Can you work these out from the model? Positions are in its coordinate system, mm. Give positions to 0.01 mm unless a question says otherwise; leave off trailing zeros. Order: outer loops, then holes, each group sorted by start corner. A loop starts at its lowest first (then second) coordinate and runs counter-clockwise, first axis right, second up.
Item 1: I'm going to push a flat-ended pin straight in: pin 1 Ø1 at (x, y) = (4, 6) entering from -Z. Where does the tip first touch, or does it pass through?
Item 2: I want a section at A-A, the plane x = 0. Write out the boundary of the cut face in (y, z), then the cut area to 3 significant figures.
Item 3: If I drill on line 1 along Y through (x, z) = (8.5, 70); line 2 along X through (y, z) = (-7.25, -12); line 3 along X through (y, z) = (-4.75, -23), over which ranges is the centre line in solid material (lowest first)?
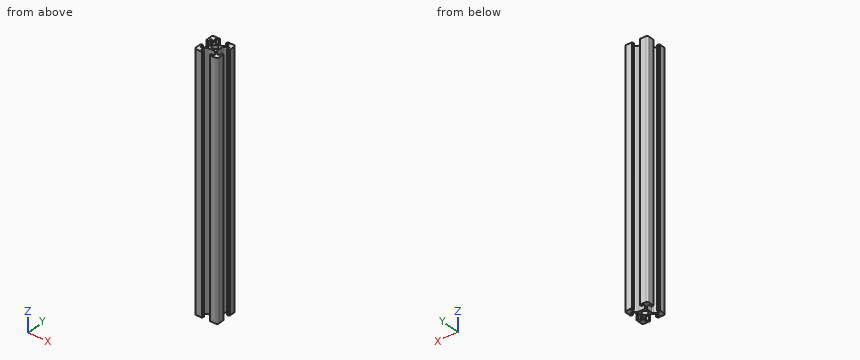
```python
from build123d import *

# Parameters (mm, degrees)
CROQUIS1_R              = 2.5
SALIENTE_EXTRUIR1_DEPTH = 110


with BuildPart() as part:
    # Croquis1 → Saliente-Extruir1 (new, symmetric)
    with BuildSketch(Plane.XY):
        with BuildLine():
            Line((-4.485786438, -3.6372583), (-6.6, -5.751471863))
            Line((-6.6, -5.751471863), (-8.2, -5.751471863))
            Line((-8.2, -5.751471863), (-8.2, -3.1))
            Line((-8.2, -3.1), (-9.5, -3.1))
            Line((-9.5, -3.1), (-9.5, -3.4))
            ThreePointArc((-9.5, -3.4), (-9.558578644, -3.541421356), (-9.7, -3.6))
            Line((-9.7, -3.6), (-10, -3.6))
            Line((-10, -3.6), (-10, -8.5))
            ThreePointArc((-10, -8.5), (-9.560660172, -9.560660172), (-8.5, -10))
            Line((-8.5, -10), (-3.6, -10))
            Line((-3.6, -10), (-3.6, -9.7))
            ThreePointArc((-3.6, -9.7), (-3.541421356, -9.558578644), (-3.4, -9.5))
            Line((-3.4, -9.5), (-3.1, -9.5))
            Line((-3.1, -9.5), (-3.1, -8.2))
            Line((-3.1, -8.2), (-5.751471863, -8.2))
            Line((-5.751471863, -8.2), (-5.751471863, -6.6))
            Line((-5.751471863, -6.6), (-3.6372583, -4.485786438))
            ThreePointArc((-3.6372583, -4.485786438), (-2.988411603, -4.052240935), (-2.223044738, -3.9))
            Line((-2.223044738, -3.9), (2.223044738, -3.9))
            ThreePointArc((2.223044738, -3.9), (2.988411603, -4.052240935), (3.6372583, -4.485786438))
            Line((3.6372583, -4.485786438), (5.751471863, -6.6))
            Line((5.751471863, -6.6), (5.751471863, -8.2))
            Line((5.751471863, -8.2), (3.1, -8.2))
            Line((3.1, -8.2), (3.1, -9.5))
            Line((3.1, -9.5), (3.4, -9.5))
            ThreePointArc((3.4, -9.5), (3.541421356, -9.558578644), (3.6, -9.7))
            Line((3.6, -9.7), (3.6, -10))
            Line((3.6, -10), (8.5, -10))
            ThreePointArc((8.5, -10), (9.560660172, -9.560660172), (10, -8.5))
            Line((10, -8.5), (10, -3.6))
            Line((10, -3.6), (9.7, -3.6))
            ThreePointArc((9.7, -3.6), (9.558578644, -3.541421356), (9.5, -3.4))
            Line((9.5, -3.4), (9.5, -3.1))
            Line((9.5, -3.1), (8.2, -3.1))
            Line((8.2, -3.1), (8.2, -5.751471863))
            Line((8.2, -5.751471863), (6.6, -5.751471863))
            Line((6.6, -5.751471863), (4.485786438, -3.6372583))
            ThreePointArc((4.485786438, -3.6372583), (4.052240935, -2.988411603), (3.9, -2.223044738))
            Line((3.9, -2.223044738), (3.9, 2.223044738))
            ThreePointArc((3.9, 2.223044738), (4.052240935, 2.988411603), (4.485786438, 3.6372583))
            Line((4.485786438, 3.6372583), (6.6, 5.751471863))
            Line((6.6, 5.751471863), (8.2, 5.751471863))
            Line((8.2, 5.751471863), (8.2, 3.1))
            Line((8.2, 3.1), (9.5, 3.1))
            Line((9.5, 3.1), (9.5, 3.4))
            ThreePointArc((9.5, 3.4), (9.558578644, 3.541421356), (9.7, 3.6))
            Line((9.7, 3.6), (10, 3.6))
            Line((10, 3.6), (10, 8.5))
            ThreePointArc((10, 8.5), (9.560660172, 9.560660172), (8.5, 10))
            Line((8.5, 10), (3.6, 10))
            Line((3.6, 10), (3.6, 9.7))
            ThreePointArc((3.6, 9.7), (3.541421356, 9.558578644), (3.4, 9.5))
            Line((3.4, 9.5), (3.1, 9.5))
            Line((3.1, 9.5), (3.1, 8.2))
            Line((3.1, 8.2), (5.751471863, 8.2))
            Line((5.751471863, 8.2), (5.751471863, 6.6))
            Line((5.751471863, 6.6), (3.6372583, 4.485786438))
            ThreePointArc((3.6372583, 4.485786438), (2.988411603, 4.052240935), (2.223044738, 3.9))
            Line((2.223044738, 3.9), (-2.223044738, 3.9))
            ThreePointArc((-2.223044738, 3.9), (-2.988411603, 4.052240935), (-3.6372583, 4.485786438))
            Line((-3.6372583, 4.485786438), (-5.751471863, 6.6))
            Line((-5.751471863, 6.6), (-5.751471863, 8.2))
            Line((-5.751471863, 8.2), (-3.1, 8.2))
            Line((-3.1, 8.2), (-3.1, 9.5))
            Line((-3.1, 9.5), (-3.4, 9.5))
            ThreePointArc((-3.4, 9.5), (-3.541421356, 9.558578644), (-3.6, 9.7))
            Line((-3.6, 9.7), (-3.6, 10))
            Line((-3.6, 10), (-8.5, 10))
            ThreePointArc((-8.5, 10), (-9.560660172, 9.560660172), (-10, 8.5))
            Line((-10, 8.5), (-10, 3.6))
            Line((-10, 3.6), (-9.7, 3.6))
            ThreePointArc((-9.7, 3.6), (-9.558578644, 3.541421356), (-9.5, 3.4))
            Line((-9.5, 3.4), (-9.5, 3.1))
            Line((-9.5, 3.1), (-8.2, 3.1))
            Line((-8.2, 3.1), (-8.2, 5.751471863))
            Line((-8.2, 5.751471863), (-6.6, 5.751471863))
            Line((-6.6, 5.751471863), (-4.485786438, 3.6372583))
            ThreePointArc((-4.485786438, 3.6372583), (-4.052240935, 2.988411603), (-3.9, 2.223044738))
            Line((-3.9, 2.223044738), (-3.9, -2.223044738))
            ThreePointArc((-3.9, -2.223044738), (-4.052240935, -2.988411603), (-4.485786438, -3.6372583))
        make_face()
        Circle(CROQUIS1_R, mode=Mode.SUBTRACT)
    extrude(amount=SALIENTE_EXTRUIR1_DEPTH, both=True)


solid = part.part
```
Results list:
1. pin 1: passes through
2. outline: (-3.9, -110) - (-2.5, -110) - (-2.5, 110) - (-3.9, 110) - close; (2.5, -110) - (3.9, -110) - (3.9, 110) - (2.5, 110) - close
2. area: 616 mm2
3. line 1: y = -10 to -3.1, 3.1 to 10
3. line 2: x = -10 to -5.75, 5.75 to 10
3. line 3: x = -10 to -8.2, -5.6 to -3.9, 3.9 to 5.6, 8.2 to 10
